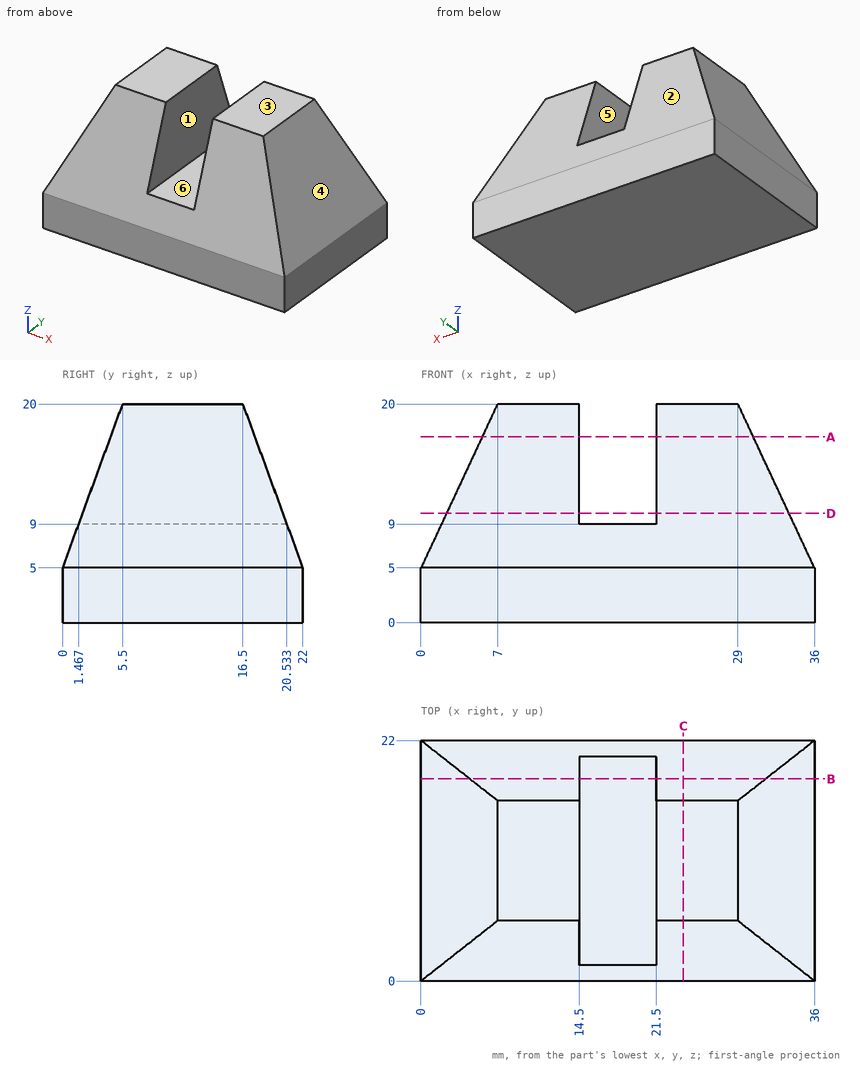
The figure shows three views and two pictorial views of one solid part (mm, origin at its lowest corner). Answer the questions. A direction names the side the tool comes from. Round coordinates to 2 decimals unless told otherwise and drop trailing zeros. Write each loop counter-clockwise with the first axis right and the second up, starting at its lowest first coordinate (ties: lowest second). Pieces come first, ordered by that corner, then holes. Notation, with made-up numbers: M 33,-37.5 L 75,-37.5 A28 cw 75,-19.5 Z; hole C 40,34.25 d9. An arc over 180 degrees is marked long. Write each question's results on one line, items separated by ' | '. Start each with the question number.
(1) The part is cut by section A-A, the plane z = 17. Write down the section's boundary in (x, y), and give its area (3 significant figures).
(2) The part is cut by section C-C, the plane x = 24. Write down the section's boundary in (y, z).
(3) For the marked faces 1 and 2, determine the directions among +Z, -Z, +X, -X, +Y, -Y from which every point of the face is accessible in a straight line to the end or side of a thin tool.
(4) Determine the mould class of the marked faces 3, 4, 5 and 6 for opening direction X: +X half, -X half, draft (parallel to the pull), parting line (faces both ways), or undercut.
(5) Each of these flat-tipped pins is pushed along its axis until it touches: P1, Ø8, axis at x = 19.5, y = 3.5, coming from the -Z side; P2, Ø5.5, axis at y = 15.5, z = 12.5, coming from the -X side; P3, Ø5.5, axis at x = 18, y = 8, coming from the +Z side; P4, Ø5.5, axis at y = 15, z = 15, coming from the +X side. Where does it stop, or does it pass through?
(6) Find the intervals of material crossed by line 1 (Z direction, x = 17.5, y = 17.75); line 2 (X direction, y = 3, z = 13); line 3 (X direction, y = 7, z = 12.5), in increasing order.
(7) The part is cut by section B-B, the plane y = 18.5. Write down the section's boundary in (x, z) (1 decimal).
(8) The part is cut by section D-D, the plane z = 10. Write down the section's boundary in (x, y), and give its area (3 significant figures).
Worked answers:
1) outline: M 5.6,4.4 L 14.5,4.4 L 14.5,17.6 L 5.6,17.6 Z; M 21.5,4.4 L 30.4,4.4 L 30.4,17.6 L 21.5,17.6 Z | area: 235 mm²
2) outline: M 0,0 L 22,0 L 22,5 L 16.5,20 L 5.5,20 L 0,5 Z
3) face 1: +Z, +Y, -Y | face 2: +Z, +X, -X, +Y
4) face 3: draft | face 4: +X half | face 5: undercut | face 6: undercut
5) P1: stops at z = 0 | P2: stops at x = 2.22 | P3: stops at z = 9 | P4: stops at x = 32.62
6) line 1: z = 0 to 9 | line 2: x = 3.73 to 14.5, 21.5 to 32.27 | line 3: x = 3.5 to 14.5, 21.5 to 32.5
7) outline: M 0,0 L 36,0 L 36,5 L 31.5,14.5 L 21.5,14.5 L 21.5,9 L 14.5,9 L 14.5,14.5 L 4.5,14.5 L 0,5 Z
8) outline: M 2.33,1.83 L 14.5,1.83 L 14.5,20.17 L 2.33,20.17 Z; M 21.5,1.83 L 33.67,1.83 L 33.67,20.17 L 21.5,20.17 Z | area: 446 mm²
